Geometry: final body of the model. Coordinates: model frame, mm. Round coordinates to 2 decimals unless told otherwise and drop trailing zeros. Write each loop counter-clockwise with the first axis right and the second up, starting at its lowest first coordinate (ties: lowest second). Pieces come first, ordered by that corner, then holes. Notation, with made-up numbers: (2.25, 28) - (18.25, 28) arc R20 ccw to (18.25, 38) - close; hole circle Ø3 at (23.5, 24). An arc over 180 degrees is marked (long way). Write each question's results on one line, items separated by ' | '.
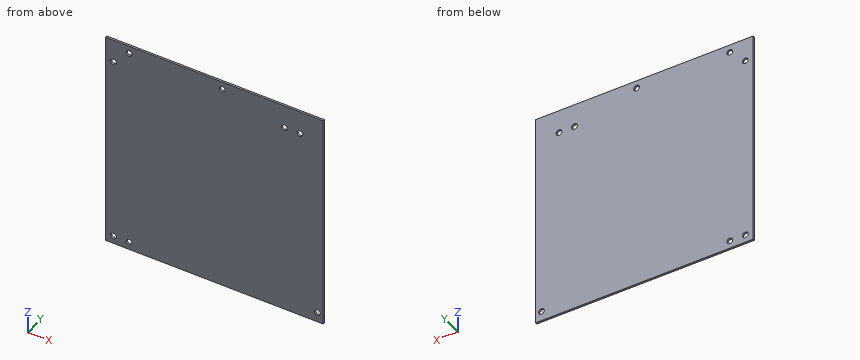
Autodesk Inventor part; units mm, degrees
ref_plane "YZ Plane" through (0, 0, 0) normal (1, 0, 0) x (0, 1, 0)
ref_plane "XZ Plane" through (0, 0, 0) normal (0, 1, 0) x (-1, 0, 0)
ref_plane "XY Plane" through (0, 0, 0) normal (0, 0, 1) x (1, 0, 0)
sketch "Sketch1" plane through (0, 0, 0) normal (0, 1, 0) x (-1, 0, 0)
  line L0 (0, 0) -> (177.8, 0)
  line L1 (177.8, 0) -> (177.8, -177.8)
  line L2 (177.8, -177.8) -> (0, -177.8)
  line L3 (0, -177.8) -> (0, 0)
  dimension "d0" = 177.8
  dimension "d1" = 177.8
extrude "Extrusion1" add sketch "Sketch1" along normal blind 1.5875
sketch "Sketch2" plane through (0, 1.5875, 0) normal (0, 1, 0) x (1, 0, 0)
  line L0 (-177.8, 177.8) -> (-177.8, 0)
  line L1 (-177.8, 177.8) -> (-177.8, 165.1)
  line L2 (-177.8, 165.1) -> (-165.1, 177.8)
  line L3 (0, 177.8) -> (-177.8, 177.8)
  line L4 (-177.8, 177.8) -> (-171.45, 171.45)
  line L5 (-171.45, 171.45) -> (-158.75, 171.45)
  line L6 (-177.8, 0) -> (-165.1, 0)
  line L7 (-177.8, 0) -> (0, 0)
  line L8 (0, 177.8) -> (-12.7, 177.8)
  line L9 (0, 0) -> (0, 177.8)
  line L10 (0, 0) -> (0, 12.7)
  line L11 (0, 12.7) -> (-12.7, 0)
  line L12 (0, 0) -> (-6.35, 6.35)
  line L13 (-6.35, 6.35) -> (-6.35, 19.05)
  line L14 (-6.35, 19.05) -> (-19.05, 19.05)
  line L15 (-19.05, 19.05) -> (-31.75, 19.05)
  line L16 (-12.7, 177.8) -> (0, 165.1)
  line L17 (0, 177.8) -> (-6.35, 171.45)
  line L18 (-165.1, 0) -> (-177.8, 12.7)
  line L19 (-177.8, 0) -> (-171.45, 6.35)
  line L20 (-171.45, 6.35) -> (-171.45, 19.05)
  line L21 (-171.45, 6.35) -> (-158.75, 6.35)
  line L22 (-6.35, 171.45) -> (-6.35, 169.799)
  line L23 (-6.35, 169.799) -> (-4.699, 169.799)
  dimension "d4" = 12.7
  dimension "d5" = 45
  dimension "d6" = 12.7
  dimension "d7" = 12.7
  dimension "d12" = 12.7
  dimension "d28" = 1.651
hole "Hole2" at (-171.45, 1.5875, -171.45) at (-158.75, 1.5875, -171.45) at (-19.05, 1.5875, -19.05) at (-31.75, 1.5875, -19.05) at (-171.45, 1.5875, -19.05) at (-158.75, 1.5875, -6.35) at (-4.699, 1.5875, -169.799) direction (0, -1, 0) diameter 4.7625 end through all
sketch "Sketch3" plane through (0, 1.5875, 0) normal (0, 1, 0) x (1, 0, 0)
  line L0 (0, 0) -> (0, 12.7)
  line L1 (0, 0) -> (0, 177.8)
  line L2 (0, 12.7) -> (-12.7, 0)
  line L3 (-177.8, 0) -> (0, 0)
  line L4 (-12.7, 0) -> (0, 0)
  line L5 (0, 0) -> (-6.35, 6.35)
  line L6 (-6.35, 6.35) -> (-82.55, 6.35)
  dimension "d29" = 12.7
  dimension "d30" = 45
  dimension "d31" = 76.2
hole "Hole3" at (-82.55, 1.5875, -6.35) direction (0, -1, 0) diameter 4.7625 end through all
properties part number "shoot" material "ABS Plastic"
Q1. Section query A-A, the plane x = -19.05. Return loops of the section in (y, z).
Answer block:
outline: (0, -177.8) - (1.59, -177.8) - (1.59, -21.43) - (0, -21.43) - close; (0, -16.67) - (1.59, -16.67) - (1.59, 0) - (0, 0) - close
Q2. Section query C-C, the plane x = -158.75. Return loops of the section in (y, z).
Answer block:
outline: (0, -177.8) - (1.59, -177.8) - (1.59, -173.83) - (0, -173.83) - close; (0, -169.07) - (1.59, -169.07) - (1.59, -8.73) - (0, -8.73) - close; (0, -3.97) - (1.59, -3.97) - (1.59, 0) - (0, 0) - close
Q3. Section query B-B, the plane z = -19.05. Return loops of the section in (x, y), plus the area to 3 significant figures.
Answer block:
outline: (-177.8, 0) - (-173.83, 0) - (-173.83, 1.59) - (-177.8, 1.59) - close; (-169.07, 0) - (-34.13, 0) - (-34.13, 1.59) - (-169.07, 1.59) - close; (-29.37, 0) - (-21.43, 0) - (-21.43, 1.59) - (-29.37, 1.59) - close; (-16.67, 0) - (0, 0) - (0, 1.59) - (-16.67, 1.59) - close | area: 260 mm2
Q4. Ray query, line 1 along X through (y, z) = (0.5, -6.35); line 2 along Z through (x, y) = (-158.75, 0.4); line 3 along X through (y, z) = (0.55, -19.05). Return the intervals inside material, ascending.
Answer block:
line 1: -177.8 to -161.13, -156.37 to -84.93, -80.17 to 0 | line 2: -177.8 to -173.83, -169.07 to -8.73, -3.97 to 0 | line 3: -177.8 to -173.83, -169.07 to -34.13, -29.37 to -21.43, -16.67 to 0
